from build123d import *

# Parameters (mm, degrees)
F0_R          = 3
F0_R_2        = 2.5
F1_DEPTH      = 460
F2_R          = 2
F3_R          = 7
F5_DEPTH      = 30
F5_DEPTH_BACK = 30


# Not quite as in the source:
# - a feature names something its author has since deleted; it is built from what else it names


with BuildPart() as f1:
    # F0 (on Top) → F1 (new body)
    with BuildSketch(Plane.XY):
        with BuildLine():
            Line((18.15, -30), (30, -30))
            Line((30, -30), (30, -18.15))
            Line((30, -18.15), (27.5, -18.15))
            Line((27.5, -18.15), (27.5, -20.15))
            Line((27.5, -20.15), (21.5477069044, -20.15))
            ThreePointArc((21.5477069044, -20.15), (19.5, -15), (21.5477069044, -9.85))
            Line((21.5477069044, -9.85), (27.5, -9.85))
            Line((27.5, -9.85), (27.5, -11.85))
            Line((27.5, -11.85), (30, -11.85))
            Line((30, -11.85), (30, 11.85))
            Line((30, 11.85), (27.5, 11.85))
            Line((27.5, 11.85), (27.5, 9.85))
            Line((27.5, 9.85), (21.5477069044, 9.85))
            ThreePointArc((21.5477069044, 9.85), (19.5, 15), (21.5477069044, 20.15))
            Line((21.5477069044, 20.15), (27.5, 20.15))
            Line((27.5, 20.15), (27.5, 18.15))
            Line((27.5, 18.15), (30, 18.15))
            Line((30, 18.15), (30, 30))
            Line((30, 30), (18.15, 30))
            Line((18.15, 30), (18.15, 27.5))
            Line((18.15, 27.5), (20.15, 27.5))
            Line((20.15, 27.5), (20.15, 21.5477069044))
            ThreePointArc((20.15, 21.5477069044), (15, 19.5), (9.85, 21.5477069044))
            Line((9.85, 21.5477069044), (9.85, 27.5))
            Line((9.85, 27.5), (11.85, 27.5))
            Line((11.85, 27.5), (11.85, 30))
            Line((11.85, 30), (-11.85, 30))
            Line((-11.85, 30), (-11.85, 27.5))
            Line((-11.85, 27.5), (-9.85, 27.5))
            Line((-9.85, 27.5), (-9.85, 21.5477069044))
            ThreePointArc((-9.85, 21.5477069044), (-15, 19.5), (-20.15, 21.5477069044))
            Line((-20.15, 21.5477069044), (-20.15, 27.5))
            Line((-20.15, 27.5), (-18.15, 27.5))
            Line((-18.15, 27.5), (-18.15, 30))
            Line((-18.15, 30), (-30, 30))
            Line((-30, 30), (-30, 18.15))
            Line((-30, 18.15), (-27.5, 18.15))
            Line((-27.5, 18.15), (-27.5, 20.15))
            Line((-27.5, 20.15), (-21.5477069044, 20.15))
            ThreePointArc((-21.5477069044, 20.15), (-19.5, 15), (-21.5477069044, 9.85))
            Line((-21.5477069044, 9.85), (-27.5, 9.85))
            Line((-27.5, 9.85), (-27.5, 11.85))
            Line((-27.5, 11.85), (-30, 11.85))
            Line((-30, 11.85), (-30, -11.85))
            Line((-30, -11.85), (-27.5, -11.85))
            Line((-27.5, -11.85), (-27.5, -9.85))
            Line((-27.5, -9.85), (-21.5477069044, -9.85))
            ThreePointArc((-21.5477069044, -9.85), (-19.5, -15), (-21.5477069044, -20.15))
            Line((-21.5477069044, -20.15), (-27.5, -20.15))
            Line((-27.5, -20.15), (-27.5, -18.15))
            Line((-27.5, -18.15), (-30, -18.15))
            Line((-30, -18.15), (-30, -30))
            Line((-30, -30), (-18.15, -30))
            Line((-18.15, -30), (-18.15, -27.5))
            Line((-18.15, -27.5), (-20.15, -27.5))
            Line((-20.15, -27.5), (-20.15, -21.5477069044))
            ThreePointArc((-20.15, -21.5477069044), (-15, -19.5), (-9.85, -21.5477069044))
            Line((-9.85, -21.5477069044), (-9.85, -27.5))
            Line((-9.85, -27.5), (-11.85, -27.5))
            Line((-11.85, -27.5), (-11.85, -30))
            Line((-11.85, -30), (11.85, -30))
            Line((11.85, -30), (11.85, -27.5))
            Line((11.85, -27.5), (9.85, -27.5))
            Line((9.85, -27.5), (9.85, -21.5477069044))
            ThreePointArc((9.85, -21.5477069044), (15, -19.5), (20.15, -21.5477069044))
            Line((20.15, -21.5477069044), (20.15, -27.5))
            Line((20.15, -27.5), (18.15, -27.5))
            Line((18.15, -27.5), (18.15, -30))
        make_face()
        with Locations((-25, -25)):
            Circle(F0_R, mode=Mode.SUBTRACT)
        with Locations((-15, -15)):
            Circle(F0_R_2, mode=Mode.SUBTRACT)
        with Locations((25, -25)):
            Circle(F0_R, mode=Mode.SUBTRACT)
        with Locations((15, -15)):
            Circle(F0_R_2, mode=Mode.SUBTRACT)
        with Locations((-25, 25)):
            Circle(F0_R, mode=Mode.SUBTRACT)
        with Locations((-15, 15)):
            Circle(F0_R_2, mode=Mode.SUBTRACT)
        Polygon((-7, 22), (-7, 27.5), (0, 27.5), (7, 27.5), (7, 22), (10, 16), (10, 10), (16, 10), (22, 7), (27.5, 7), (27.5, 0), (27.5, -7), (22, -7), (16, -10), (10, -10), (10, -16), (7, -22), (7, -27.5), (0, -27.5), (-7, -27.5), (-7, -22), (-10, -16), (-10, -10), (-16, -10), (-22, -7), (-27.5, -7), (-27.5, 0), (-27.5, 7), (-22, 7), (-16, 10), (-10, 10), (-10, 16), align=None, mode=Mode.SUBTRACT)
        with Locations((15, 15)):
            Circle(F0_R_2, mode=Mode.SUBTRACT)
        with Locations((25, 25)):
            Circle(F0_R, mode=Mode.SUBTRACT)
    extrude(amount=F1_DEPTH)

    # F2
    f2_edges = [f1.edges().sort_by_distance(p)[0] for p in [
        (-7, 27.5, 230),
        (7, 27.5, 230),
    ]]
    fillet(f2_edges, radius=F2_R)

    # F3
    f3_edges = [f1.edges().sort_by_distance(p)[0] for p in [
        (-10, 16, 230),
        (10, 16, 230),
    ]]
    fillet(f3_edges, radius=F3_R)

    # F4 (on Right) → F5 (cut, two sides)
    with BuildSketch(Plane.YZ) as f5_sk:
        Polygon((30, 460), (-101.7983138763, 778.1892768581), (-315.3200388241, 689.7456825234), (-183.5217249478, 371.5564056653), align=None)
    extrude(amount=F5_DEPTH, mode=Mode.SUBTRACT)
    extrude(f5_sk.sketch, amount=-F5_DEPTH_BACK, mode=Mode.SUBTRACT)


solid = f1.part
Verification items for the finished model (mm, model axes). A direction names the side the tool comes from. Round coordinates to 2 decimals unless told otherwise and drop trailing zeros. Answer in a Markdown table with one row per item. Add a question column.
Q1. Material ranges on line 1 (X direction, y = 15, z = 360); line 2 (Y direction, x = 25.5, z = 350); line 3 (Y direction, x = -15, z = 270.5), recorded low to high.
Q2. Release check for a two-part mould opening along X. For faces 3 (the face through (0, 30, 227)), 4 (the face through (-30, -24, 217)), 5 (the face through (-15.1, -19.5, 216.7)), 6 (the face through (30, 0, 223)) record: pulls with the +X half, pulls with the -X half, needs draft (parallel to the pull), parting line crosses it, or undercut.
Q3. Gauge pin test, flat ends, axial feed: pin 1 (1 mm diameter, centred on y = 15, z = 380, fed in from -X); pin 2 (8 mm diameter, centred on x = -23, y = -23.5, fed in from +Z). Record the tip position at first contact, or that the pin passes through.
Q4. Section check A-A on z = 36.5. State how many separate pieces and enclosed holes the cut face has, plus the area to 3 significant figures.
Q5. Tool access check on faces 1 (the face through (-19.5, -14.9, 218.6)), 2 (the face through (-30, 0, 223)). Record the directions out of +Z, -Z, +X, -X, +Y, -Y that give a thin tool (end or side, any length) a straight path to the whole face; none if there is none.
Found:
| question | item | result |
|---|---|---|
| 1 | line 1 | x = -19.5 to -17.5, -12.5 to -9.97, 9.97 to 12.5, 17.5 to 19.5 |
| 1 | line 2 | y = -30 to -27.96, -22.04 to -20.15, -9.85 to -7, 7 to 9.85, 20.15 to 22.04, 27.96 to 30 |
| 1 | line 3 | y = -19.5 to -17.5, -12.5 to -10, 10 to 12.5, 17.5 to 19.5 |
| 2 | face 3 | needs draft |
| 2 | face 4 | pulls with the -X half |
| 2 | face 5 | undercut |
| 2 | face 6 | pulls with the +X half |
| 3 | pin 1 | stops at x = -19.52 |
| 3 | pin 2 | stops at z = 439.34 |
| 4 | separate pieces | 1 |
| 4 | enclosed holes | 9 |
| 4 | area | 1,080 mm² |
| 5 | face 1 | +Z, -Z |
| 5 | face 2 | +Z, -Z, -X, +Y, -Y |
